```python
from build123d import *

# Parameters (mm, degrees)
BOSS_EXTRUDE1_DEPTH     = 2.25
BOSS_EXTRUDE2_START     = 2.25
SKETCH1_4_R             = 3.25
BOSS_EXTRUDE2_DEPTH     = 2
BOSS_EXTRUDE3_START     = 4.25
BOSS_EXTRUDE3_DEPTH     = 2
BOSS_EXTRUDE6_DEPTH     = 33.8
BOSS_EXTRUDE7_DEPTH     = 3.8
FILLET1_R               = 2
FILLET2_R               = 2
FILLET3_R               = 0.5
CUT_EXTRUDE1_REACH      = 54.552
CUT_EXTRUDE1_END_RADIUS = 27.541666667
SKETCH6_R               = 3.25


with BuildPart() as part:
    # Sketch1 → Boss-Extrude1 (new body)
    with BuildSketch(Plane(origin=(0, 0, 0), x_dir=(1, 0, 0), z_dir=(0, 1, 0))):
        with BuildLine():
            Line((30, -12.5), (30, 12.5))
            Line((30, 12.5), (0, 12.5))
            Line((0, 12.5), (0, 9.25))
            ThreePointArc((0, 9.25), (9.25, 0), (0, -9.25))
            Line((0, -9.25), (0, -12.5))
            Line((0, -12.5), (30, -12.5))
        make_face()
    extrude(amount=BOSS_EXTRUDE1_DEPTH)

    # Sketch1<4> → Boss-Extrude2 (add)
    with BuildSketch(Plane(origin=(0, 0, 0), x_dir=(1, 0, 0), z_dir=(0, 1, 0)).offset(BOSS_EXTRUDE2_START)):
        with BuildLine():
            Line((30, -12.5), (30, 12.5))
            Line((30, 12.5), (0, 12.5))
            Line((0, 12.5), (0, 8.25))
            ThreePointArc((0, 8.25), (-8.25, 0), (0, -8.25))
            Line((0, -8.25), (0, -12.5))
            Line((0, -12.5), (30, -12.5))
        make_face()
        with Locations(Location((0, 0, 0), (0, 0, 270))):
            Circle(SKETCH1_4_R, mode=Mode.SUBTRACT)
    extrude(amount=BOSS_EXTRUDE2_DEPTH)

    # Sketch1<6> → Boss-Extrude3 (add)
    with BuildSketch(Plane(origin=(0, 0, 0), x_dir=(1, 0, 0), z_dir=(0, 1, 0)).offset(BOSS_EXTRUDE3_START)):
        with BuildLine():
            Line((0, -12.5), (22, -12.5))
            ThreePointArc((22, -12.5), (19, 0), (22, 12.5))
            Line((22, 12.5), (0, 12.5))
            Line((0, 12.5), (0, 9.25))
            ThreePointArc((0, 9.25), (9.25, 0), (0, -9.25))
            Line((0, -9.25), (0, -12.5))
        make_face()
        with BuildLine():
            Line((22, -12.5), (30, -12.5))
            Line((30, -12.5), (30, 12.5))
            Line((30, 12.5), (22, 12.5))
            ThreePointArc((22, 12.5), (19, 0), (22, -12.5))
        make_face()
    extrude(amount=BOSS_EXTRUDE3_DEPTH)

    # Sketch1<8> → Boss-Extrude6 (add)
    with BuildSketch(Plane(origin=(0, 0, 0), x_dir=(1, 0, 0), z_dir=(0, 1, 0))):
        with BuildLine():
            Line((22, -12.5), (30, -12.5))
            Line((30, -12.5), (30, 12.5))
            Line((30, 12.5), (22, 12.5))
            ThreePointArc((22, 12.5), (19, 0), (22, -12.5))
        make_face()
    extrude(amount=BOSS_EXTRUDE6_DEPTH)

    # Sketch3 → Boss-Extrude7 (add)
    with BuildSketch(Plane(origin=(0, 33.8, 0), x_dir=(1, 0, 0), z_dir=(0, 1, 0))):
        with BuildLine():
            Line((11, 0), (19, 0))
            ThreePointArc((19, 0), (19.473969858, 5.087552676), (20.879566153, 10))
            Line((20.879566153, 10), (11, 0))
        make_face()
        with BuildLine():
            ThreePointArc((20.879566153, -10), (19.473969858, -5.087552676), (19, 0))
            Line((19, 0), (11, 0))
            Line((11, 0), (20.879566153, -10))
        make_face()
        with BuildLine():
            ThreePointArc((20.879566153, 10), (19.473969858, 5.087552676), (19, 0))
            ThreePointArc((19, 0), (19.473969858, -5.087552676), (20.879566153, -10))
            ThreePointArc((20.879566153, -10), (21.408679185, -11.263939941), (22, -12.5))
            Line((22, -12.5), (30, -12.5))
            Line((30, -12.5), (30, 12.5))
            Line((30, 12.5), (22, 12.5))
            ThreePointArc((22, 12.5), (21.408679185, 11.263939941), (20.879566153, 10))
        make_face()
    extrude(amount=-BOSS_EXTRUDE7_DEPTH)

    # Fillet1
    fillet1_edges = [part.edges().sort_by_distance(p)[0] for p in [
        (11, 31.9, 0),
    ]]
    fillet(fillet1_edges, radius=FILLET1_R)

    # Fillet2
    fillet2_edges = [part.edges().sort_by_distance(p)[0] for p in [
        (30, 16.9, -12.5),
        (30, 16.9, 12.5),
        (22, 20.025, -12.5),
        (22, 20.025, 12.5),
    ]]
    fillet(fillet2_edges, radius=FILLET2_R)

    # Fillet3
    fillet3_edges = [part.edges().sort_by_distance(p)[0] for p in [
        (0, 1.125, 9.25),
        (0, 1.125, -9.25),
        (0, 2.25, -8.75),
        (0, 2.25, 8.75),
        (-8.25, 4.25, 0),
        (0, 4.25, 8.75),
        (-8.25, 2.25, 0),
        (0, 4.25, -8.75),
        (0, 5.25, -9.25),
        (0, 5.25, 9.25),
    ]]
    fillet(fillet3_edges, radius=FILLET3_R)

    # Cut-Extrude1: up to this cylinder (the profile starts inside it)
    cut_extrude1_end = Plane(origin=(46.541666667, 23, 0), z_dir=(0, -1, 0)) * Cylinder(CUT_EXTRUDE1_END_RADIUS, 165.187333333, mode=Mode.PRIVATE)
    # Sketch6 → Cut-Extrude1 (cut, up to the surface)
    with BuildSketch(Plane(origin=(30, 0, 0), x_dir=(0, 0, -1), z_dir=(1, 0, 0)), mode=Mode.PRIVATE) as cut_extrude1_sk1:
        with Locations((0, 23)):
            Circle(SKETCH6_R)
    cut_extrude1_tool1 = extrude(cut_extrude1_sk1.sketch, amount=-CUT_EXTRUDE1_REACH, mode=Mode.PRIVATE) & cut_extrude1_end
    add(cut_extrude1_tool1.solids().sort_by_distance((30, 23, 0))[0], mode=Mode.SUBTRACT)


solid = part.part
```
Check sheet for the modelled part. Datum: model origin and axes. Units: mm. A direction names the side the tool comes from. Coordinates: 2 decimals unless noted, no trailing zeros. Order: outer loops, then holes, each group sorted by start corner. A loop starts at its lowest first (then second) coordinate and runs counter-clockwise, first axis right, second up. Notation, with made-up numbers: (59, -25.5) -> (101, -25.5) arc R14 ccw to (101, -0.5) -> close; hole circle Ø1 at (24, -35). An arc over 180 degrees is marked (long way). Write each question's results on one line, items separated by ' | '. Start each with the question number.
1) Section check D-D (y = 23). Enter the section's corners in (x, z).
2) Draft check along Y on faces 1 (the face through (24.575, 19.827, 0.705)), 2 (the face through (18, 0, 0)), 3 (the face through (-8.25, 3.24, -0.18)). Enter one of: pulls with the +Y half, pulls with the -Y half, needs draft (parallel to the pull), parting line crosses it, or undercut.
3) Depth check by flat-ended pin: pin 1 (5 mm diameter, centred on x = 4.5, z = 2.5, fed in from -Y); pin 2 (7.5 mm diameter, centred on x = 17.5, z = -1, fed in from -Y); pin 3 (1 mm diameter, centred on y = 10.5, z = -7.5, fed in from -X); pin 4 (5 mm diameter, centred on x = -1.5, z = -0.5, fed in from +Y). Enter the tip coordinate at first touch or a pass-through.
4) Material ranges on line 1 along X through (y, z) = (3.8, 0); line 2 along Y through (x, z) = (28, 0); line 3 along Y through (x, z) = (15, 2.25), recorded low to high.
5) Set-up check for faces 4 (the face through (9.248, 1.11, -0.197)), 5 (the face through (3, 4.25, -2)), 6 (the face through (22.16, 19.83, -12.17)): record each of +Z, -Z, +X, -X, +Y, -Y from which the full face is reachable in a straight line by a thin tool's end or side.
6) Section check C-C (z = 0). Enter the section's corners in (x, y), and give its area (3 significant figures).
7) Section check A-A (y = 12). Enter the section's corners in (x, z).
8) Section check B-B (x = 18). Enter the section's corners in (y, z), and give its area (3 significant figures).
Checked values:
1) outline: (19.19, -3.25) arc R27.54 ccw to (21.43, -11.32) arc R2 ccw to (23.26, -12.5) -> (28, -12.5) arc R2 ccw to (30, -10.5) -> (30, -3.25) -> close; (19.19, 3.25) -> (30, 3.25) -> (30, 10.5) arc R2 ccw to (28, 12.5) -> (23.26, 12.5) arc R2 ccw to (21.43, 11.32) arc R27.54 ccw to start
2) face 1: undercut | face 2: pulls with the -Y half | face 3: needs draft
3) pin 1: y = 2.25 | pin 2: y = 0 | pin 3: x = 19.9 | pin 4: y = 4.25
4) line 1: -8.25 to -3.25, 3.25 to 30 | line 2: 0 to 19.75, 26.25 to 33.8 | line 3: 0 to 6.25, 30 to 33.8
5) face 4: -X, -Y | face 5: -X, +Y | face 6: -Z, -X, +Y
6) outline: (-8.25, 2.75) arc R0.5 ccw to (-7.75, 2.25) -> (-3.25, 2.25) -> (-3.25, 4.25) -> (-7.75, 4.25) arc R0.5 ccw to (-8.25, 3.75) -> close; (3.25, 2.25) -> (9.25, 2.25) -> (9.25, 0) -> (30, 0) -> (30, 19.75) -> (19, 19.75) -> (19, 6.25) -> (9.25, 6.25) -> (9.25, 4.25) -> (3.25, 4.25) -> close; (11.81, 30) -> (19, 30) -> (19, 26.25) -> (30, 26.25) -> (30, 33.8) -> (11.81, 33.8) -> close | area: 410 mm²
7) outline: (21.43, -11.32) arc R2 ccw to (23.26, -12.5) -> (28, -12.5) arc R2 ccw to (30, -10.5) -> (30, 10.5) arc R2 ccw to (28, 12.5) -> (23.26, 12.5) arc R2 ccw to (21.43, 11.32) arc R27.54 ccw to start
8) outline: (0, -12.5) -> (6.25, -12.5) -> (6.25, 12.5) -> (0, 12.5) -> close; (30, -7.09) -> (33.8, -7.09) -> (33.8, 7.09) -> (30, 7.09) -> close | area: 210 mm²
